Can you work these out from the model? Positions are in its coordinate system, mm. Round coordinates to 2 decimals unless told otherwise and drop trailing zeros. Write each loop counter-clockwise with the first axis right and the second up, starting at its lowest first coordinate (ties: lowest second). Pieces come first, ordered by that corner, then holes.
Q1. If we section it at A-A (y = 132.08): Please give me the cut outline in (x, z) (3 decimals), plus the area to 3 significant figures.
Q2. I'm going to push a flat-ended pin straight in: pin 1 Ø3.5 at (x, y) = (0, 154.92) entering from +Z. Where does the tip first touch, or does it pass through?
Q3. If we section it at C-C (y = 0): Please give me the cut outline in (x, z) (3 decimals).
Q4. If we section it at B-B (x = 0): Please give me the cut outline in (y, z) (3 decimals).
Q5. We'd pull the mould along Y, two halves only. Please class faces 1 (the cylindrical face through (-0.257, 156.878, -0.776)), 2 (the cylindrical face through (155.507, 0.087, -0.776)), 3 (the flat face through (78, 81, 0)): +Y half, -Y half, draft (parallel to the pull), parting line (faces both ways), or undercut.
Q6. Please list where these lines run through material, in increasing order: line 1 along X through (y, z) = (132.08, -0.35) (3 decimals); line 2 along X through (y, z) = (154.92, -0.35) (3 decimals).
from build123d import *

# Parameters (mm, degrees)
SALIENTE_EXTRUIR1_DEPTH = 1.575
CROQUIS2_R              = 1.975
CORTAR_EXTRUIR1_DEPTH   = 10


with BuildPart() as part:
    # Croquis1 → Saliente-Extruir1 (new body)
    with BuildSketch(Plane.XY):
        with BuildLine():
            Line((161.83, 165.1), (-4.35, 165.1))
            ThreePointArc((-4.35, 165.1), (-5.764213562, 164.514213562), (-6.35, 163.1))
            Line((-6.35, 163.1), (-6.35, -3.08))
            ThreePointArc((-6.35, -3.08), (-5.764213562, -4.494213562), (-4.35, -5.08))
            Line((-4.35, -5.08), (161.83, -5.08))
            ThreePointArc((161.83, -5.08), (163.244213562, -4.494213562), (163.83, -3.08))
            Line((163.83, -3.08), (163.83, 163.1))
            ThreePointArc((163.83, 163.1), (163.244213562, 164.514213562), (161.83, 165.1))
        make_face()
    extrude(amount=-SALIENTE_EXTRUIR1_DEPTH)

    # Croquis2 → Cortar-Extruir1 (cut)
    with BuildSketch(Plane.XY):
        Circle(CROQUIS2_R)
        with Locations((157.48, 0)):
            Circle(CROQUIS2_R)
        with Locations((157.48, 132.08)):
            Circle(CROQUIS2_R)
        with Locations((0, 154.919999989)):
            Circle(CROQUIS2_R)
    extrude(amount=-CORTAR_EXTRUIR1_DEPTH, mode=Mode.SUBTRACT)


solid = part.part
A:
1. outline: (-6.35, -1.575) - (155.505, -1.575) - (155.505, 0) - (-6.35, 0) - close; (159.455, -1.575) - (163.83, -1.575) - (163.83, 0) - (159.455, 0) - close
1. area: 262 mm2
2. pin 1: passes through
3. outline: (-6.35, -1.575) - (-1.975, -1.575) - (-1.975, 0) - (-6.35, 0) - close; (1.975, -1.575) - (155.505, -1.575) - (155.505, 0) - (1.975, 0) - close; (159.455, -1.575) - (163.83, -1.575) - (163.83, 0) - (159.455, 0) - close
4. outline: (-5.08, -1.575) - (-1.975, -1.575) - (-1.975, 0) - (-5.08, 0) - close; (1.975, -1.575) - (152.945, -1.575) - (152.945, 0) - (1.975, 0) - close; (156.895, -1.575) - (165.1, -1.575) - (165.1, 0) - (156.895, 0) - close
5. face 1: undercut
5. face 2: undercut
5. face 3: draft
6. line 1: x = -6.35 to 155.505, 159.455 to 163.83
6. line 2: x = -6.35 to -1.975, 1.975 to 163.83
